Source: CAD feature listing. Evaluate the final solid. Frame: model axes, mm. Face numbers are marked on the shaded views. Give positions to 0.01 mm unless a question says otherwise; leave off trailing zeros. Order: outer loops, then holes, each group sorted by start corner. A loop starts at its lowest first (then second) coordinate and runs counter-clockwise, first axis right, second up. Notation, with made-up numbers: (6, 22.5) -> (40, 22.5) arc R22 ccw to (40, 56.5) -> close; hole circle Ø1 at (57.25, 51.25). An arc over 180 degrees is marked (long way). Use one line per item in the form item = value. Start each with the question number.
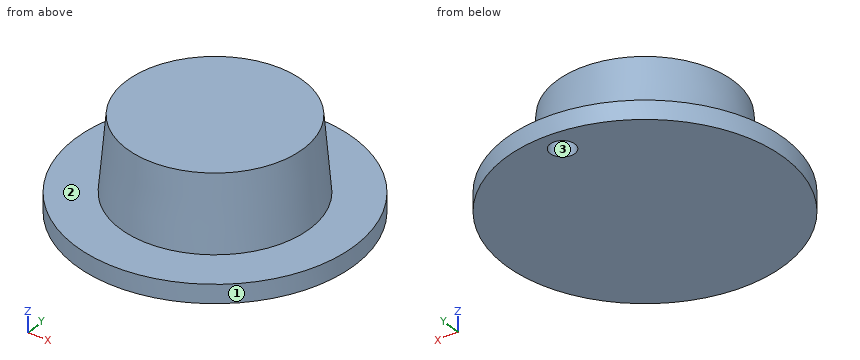
from build123d import *

# Parameters (mm, degrees)
F0_R     = 22.5
F0_R_2   = 15.3
F1_DEPTH = 3
F2_R     = 15.3
F3_DEPTH = 12
F3_TAPER = 5
F4_R     = 2
F5_DEPTH = 32.3


with BuildPart() as f1:
    # F0 (on Top) → F1 (new body)
    with BuildSketch(Plane.XY):
        Circle(F0_R)
        Circle(F0_R_2, mode=Mode.SUBTRACT)
        Circle(F0_R_2)
    extrude(amount=F1_DEPTH)

    # F2 (on face) → F3 (join)
    with BuildSketch(Plane.XY.offset(3)):
        Circle(F2_R)
    extrude(amount=F3_DEPTH, taper=F3_TAPER)

    # F4 (on face) → F5 (cut)
    with BuildSketch(Plane.XY.offset(3)):
        with Locations((0, 18.7446177006)):
            Circle(F4_R)
    extrude(amount=-F5_DEPTH, mode=Mode.SUBTRACT)


solid = f1.part
1) Pin query (flat end, axial travel): pin 1 (4 mm diameter, centred on x = -2, z = 5.5, fed in from +Y); pin 2 (1 mm diameter, centred on x = 12, y = 12.5, fed in from +Z); pin 3 (2 mm diameter, centred on x = -3, z = 9.5, fed in from -Y). Return the tip coordinate at first contact, or that it passes through.
2) Material intervals for probe 1 along Y at (x, z) = (0, 2.35); probe 2 along Z at (x, y) = (13, -15.5); probe 3 along X at (y, z) = (4.5, 10.5), sorted ascending.
3) Cut plane D-D, the plane z = 7.5. Return the cut outline in (x, y), plus the area to 3 significant figures.
4) Cut plane C-C, the plane z = 1.25. Return the cut outline in (x, y), plus the area to 3 significant figures.
5) Cut plane A-A, the plane x = 0. Return the cut outline in (y, z).
6) Draft query along X for the marked faces 1, 2 and 3. Return one class per face: +X half, -X half, draft (parallel to the pull), parting line (faces both ways), or undercut.
7) Cut plane B-B, the plane y = 0. Return the cut outline in (x, z), plus the area to 3 significant figures.
Output values:
q1.pin_1 = 15.2
q1.pin_2 = 3
q1.pin_3 = -14.62
q2.probe_1 = -22.5 to 16.74, 20.74 to 22.5
q2.probe_2 = 0 to 3
q2.probe_3 = -13.94 to 13.94
q3.outline = circle Ø29.81 at (0, 0)
q3.area = 698 mm^2
q4.outline = circle Ø45 at (0, 0); hole circle Ø4 at (0, 18.74)
q4.area = 1,580 mm^2
q5.outline = (-22.5, 0) -> (16.74, 0) -> (16.74, 3) -> (15.3, 3) -> (14.25, 15) -> (-14.25, 15) -> (-15.3, 3) -> (-22.5, 3) -> close; (20.74, 0) -> (22.5, 0) -> (22.5, 3) -> (20.74, 3) -> close
q6.face_1 = parting line
q6.face_2 = draft
q6.face_3 = undercut
q7.outline = (-22.5, 0) -> (22.5, 0) -> (22.5, 3) -> (15.3, 3) -> (14.25, 15) -> (-14.25, 15) -> (-15.3, 3) -> (-22.5, 3) -> close
q7.area = 490 mm^2
